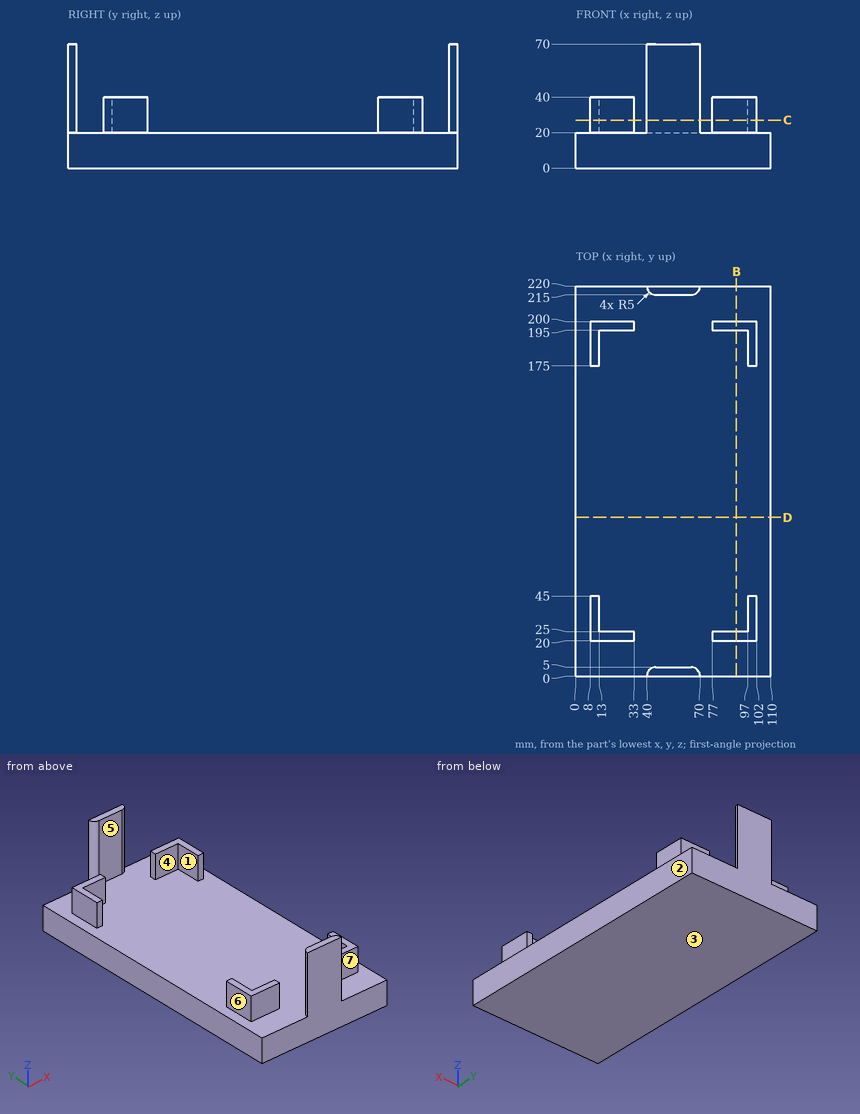
Geometry check sheet. Reference: drawing and pictorial views, mm from the part's lowest x, y, z. A direction names the side the tool comes from. Give positions to 0.01 mm unless a question says otherwise; leave off trailing zeros. Order: outer loops, then holes, each group sorted by start corner. A loop starts at its lowest first (then second) coordinate and runs counter-clockwise, first axis right, second up. Notation, with made-up numbers: (52, 54.25) -> (93, 54.25) arc R18 cw to (93, 64.25) -> close; hole circle Ø7 at (84.5, 62.25). An arc over 180 degrees is marked (long way). Use CSV: the item, a comma, the result in double quotes. Start each with the question number.
1) Material ranges on line 1 (Y direction, x = 18, z = 23); line 2 (Z direction, x = 85.5, y = 115.5); line 3 (Y direction, x = 52.5, z = 36), recorded low to high. Write a range as from..to.
2) Sectioned sample at B-B, the plane x = 90.5. Record the boundary of the cut face in (y, z), plus the area to 3 significant figures.
3) Sectioned sample at D-D, the plane y = 89.5. Record the boundary of the cut face in (x, z).
4) Go/stop test with flat-tipped pins: P1, Ø5.5, axis at x = 98.5, z = 26.5, coming from the -Y side; P2, Ø4, axis at x = 99, z = 26.5, coming from the +Y side; P3, Ø1.5, axis at y = 22, z = 34.5, coming from the -X side. Record where each tip stops, or that it passes through.
5) Mould release check, pull along X, two halves, no side actions. Record for the marked faces 1, 2, 3 and 4: released by +X, released by -X, zero draft, split by the parting line, or undercut.
6) Set-up check for the marked faces 5, 6 and 7: record each of +Z, -Z, +X, -X, +Y, -Y from which the full face is reachable in a straight line by a thin tool's end or side.
7) Sectioned sample at C-C, the plane z = 27. Give the number of separate pieces and of enclosed holes in the cut face, plus the area to 3 significant figures.
Recorded:
1,line 1,"20..25, 195..200"
1,line 2,"0..20"
1,line 3,"0..5, 215..220"
2,outline,"(0, 0) -> (220, 0) -> (220, 20) -> (200, 20) -> (200, 40) -> (195, 40) -> (195, 20) -> (25, 20) -> (25, 40) -> (20, 40) -> (20, 20) -> (0, 20) -> close"
2,area,"4,600 mm2"
3,outline,"(0, 0) -> (110, 0) -> (110, 20) -> (0, 20) -> close"
4,P1,"y = 20"
4,P2,"y = 200"
4,P3,"x = 8"
5,face 1,"undercut"
5,face 2,"released by +X"
5,face 3,"zero draft"
5,face 4,"undercut"
6,face 5,"+Z, +X, -X"
6,face 6,"+Z, -X, +Y, -Y"
6,face 7,"+Z, +X, -X, -Y"
7,separate pieces,"6"
7,enclosed holes,"0"
7,area,"1,180 mm2"
